The model under review builds one solid part; all positions refer to its coordinate system, in mm. Coordinates: 2 decimals unless noted, no trailing zeros. Order: outer loops, then holes, each group sorted by start corner. A loop starts at its lowest first (then second) coordinate and runs counter-clockwise, first axis right, second up.
from build123d import *

# Parameters (mm, degrees)
SKETCH_2_W               = 250
SKETCH_2_H               = 75
EXTRUDE_3_DEPTH          = 2
CUT_EXTRUDE_1_DEPTH      = 2
CUT_EXTRUDE_1_DEPTH_BACK = 2
SKETCH_4_W               = 2
SKETCH_4_H               = 50


with BuildPart() as part:
    # 草图2 → 凸台-拉伸3 (new body)
    with BuildSketch(Plane.XY):
        with Locations((51.318241286, 40.884671024)):
            Rectangle(SKETCH_2_W, SKETCH_2_H)
    extrude(amount=EXTRUDE_3_DEPTH)

    # 草图4 → 切除-拉伸1 (cut, two sides: drawn at the far end of the back side and taken through both)
    with BuildSketch(Plane.XY.offset(-CUT_EXTRUDE_1_DEPTH_BACK)):
        with Locations((151.318241286, 40.884671024)):
            Rectangle(SKETCH_4_W, SKETCH_4_H)
        with Locations((-48.681758714, 40.884671024)):
            Rectangle(SKETCH_4_W, SKETCH_4_H)
        with Locations((51.318241286, 40.884671024)):
            Rectangle(SKETCH_4_W, SKETCH_4_H)
    extrude(amount=CUT_EXTRUDE_1_DEPTH + CUT_EXTRUDE_1_DEPTH_BACK, mode=Mode.SUBTRACT)


solid = part.part
(1) Consider section A-A (z = 0.7). Give the boundary of the cut face in (x, y), then the cut area to 4 significant figures.
(2) Wall thickness on line 1 (X direction, y = 38, z = 0.7): over which ranges is the line inside the solid? List them lowest first.
(3) Consider section B-B (y = 53). Give the boundary of the cut face in (x, z), then the cut area to 3 significant figures.
Findings:
1. outline: (-73.68, 3.38) - (176.32, 3.38) - (176.32, 78.38) - (-73.68, 78.38) - close; hole (-49.68, 15.88) - (-47.68, 15.88) - (-47.68, 65.88) - (-49.68, 65.88) - close; hole (50.32, 15.88) - (52.32, 15.88) - (52.32, 65.88) - (50.32, 65.88) - close; hole (150.32, 15.88) - (152.32, 15.88) - (152.32, 65.88) - (150.32, 65.88) - close
1. area: 18,450 mm2
2. line 1: x = -73.68 to -49.68, -47.68 to 50.32, 52.32 to 150.32, 152.32 to 176.32
3. outline: (-73.68, 0) - (-49.68, 0) - (-49.68, 2) - (-73.68, 2) - close; (-47.68, 0) - (50.32, 0) - (50.32, 2) - (-47.68, 2) - close; (52.32, 0) - (150.32, 0) - (150.32, 2) - (52.32, 2) - close; (152.32, 0) - (176.32, 0) - (176.32, 2) - (152.32, 2) - close
3. area: 488 mm2
